Verification items for the finished model (mm, model axes). Face numbers are marked on the shaded views. A direction names the side the tool comes from. Give positions to 0.01 mm unless a question says otherwise; leave off trailing zeros. Write each loop counter-clockwise with the first axis right and the second up, starting at its lowest first coordinate (ties: lowest second). Pieces come first, ordered by that corner, then holes. Notation, with made-up numbers: M -8.75,-37.75 L 44.25,-37.75 A12 cw 44.25,-24.75 Z; hole C 6,-17.75 d11. An arc over 180 degrees is marked long. Answer as a JSON object with one key per item and string values.
```python
from build123d import *

# Parameters (mm, degrees)
SKETCH1_R                      = 6
BOSS_EXTRUDE1_DEPTH            = 2
SKETCH2_R                      = 3.95
BOSS_EXTRUDE2_DEPTH            = 7.9
CHAMFER1_SIZE                  = 0.4
CBORE_FOR_M3_SHCS1_D           = 3.2
CBORE_FOR_M3_SHCS1_CBORE_D     = 6
CBORE_FOR_M3_SHCS1_CBORE_DEPTH = 2.5


with BuildPart() as part:
    # Sketch1 → Boss-Extrude1 (new body)
    with BuildSketch(Plane(origin=(0, 0, 0), x_dir=(1, 0, 0), z_dir=(0, 1, 0))):
        Circle(SKETCH1_R)
    extrude(amount=BOSS_EXTRUDE1_DEPTH)

    # Sketch2 → Boss-Extrude2 (add)
    with BuildSketch(Plane(origin=(0, 2, 0), x_dir=(1, 0, 0), z_dir=(0, 1, 0))):
        Circle(SKETCH2_R)
    extrude(amount=BOSS_EXTRUDE2_DEPTH)

    # Chamfer1
    chamfer1_edges = [part.edges().sort_by_distance(p)[0] for p in [
        (-6, 0, 0),
        (-6, 2, 0),
        (-3.95, 9.9, 0),
    ]]
    chamfer(chamfer1_edges, length=CHAMFER1_SIZE)

    # CBORE for M3 SHCS1 (through all)
    with Locations(Plane(origin=(0, 0, 0), x_dir=(-1, 0, 0), z_dir=(0, -1, 0))):
        with Locations((0, 0)):
            CounterBoreHole(CBORE_FOR_M3_SHCS1_D / 2, CBORE_FOR_M3_SHCS1_CBORE_D / 2, CBORE_FOR_M3_SHCS1_CBORE_DEPTH)


solid = part.part
```
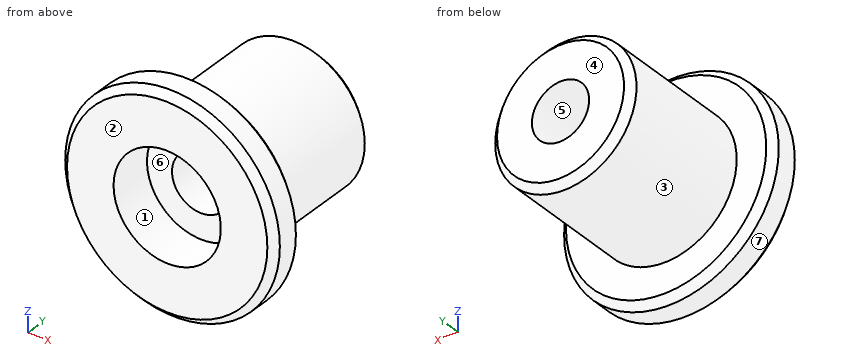
1) Access from +Z, -Z, +X, -X, +Y, -Y to the whole of each face (thin tool, end or side, straight path). Record for the marked faces 1, 2 and 3.
Completed:
{"face 1": "-Y", "face 2": "+Z, -Z, +X, -X, -Y", "face 3": "+Y"}
2) Section check D-D on y = 1.25. Record the boundary of the cut face in (x, z), and give its area (3 significant figures).
Completed:
{"outline": "C 0,0 d12; hole C 0,0 d6", "area": "84.8 mm2"}
3) Go/stop test with flat-tipped pins: pin 1 (2 mm diameter, centred on x = -4.5, y = 5.5, fed in from +Z); pin 2 (5 mm diameter, centred on y = 5.5, z = -1.5, fed in from +X); pin 3 (3 mm diameter, centred on x = -1, y = 6.5, fed in from -Z). Record where each tip stops, or that it passes through.
Completed:
{"pin 1": "stops at z = 1.83", "pin 2": "stops at x = 3.95", "pin 3": "stops at z = -3.95"}
4) Section check A-A on x = 0. Record the boundary of the cut face in (y, z).
Completed:
{"outline": "M 0,-5.6 L 0.4,-6 L 1.6,-6 L 2,-5.6 L 2,-3.95 L 9.5,-3.95 L 9.9,-3.55 L 9.9,-1.6 L 2.5,-1.6 L 2.5,-3 L 0,-3 Z; M 0,3 L 2.5,3 L 2.5,1.6 L 9.9,1.6 L 9.9,3.55 L 9.5,3.95 L 2,3.95 L 2,5.6 L 1.6,6 L 0.4,6 L 0,5.6 Z"}
5) Section check C-C on y = 5. Record the boundary of the cut face in (x, z).
Completed:
{"outline": "C 0,0 d7.9; hole C 0,0 d3.2"}
6) Section check B-B on z = 0. Record the boundary of the cut face in (x, y).
Completed:
{"outline": "M -6,0.4 L -5.6,0 L -3,0 L -3,2.5 L -1.6,2.5 L -1.6,9.9 L -3.55,9.9 L -3.95,9.5 L -3.95,2 L -5.6,2 L -6,1.6 Z; M 1.6,2.5 L 3,2.5 L 3,0 L 5.6,0 L 6,0.4 L 6,1.6 L 5.6,2 L 3.95,2 L 3.95,9.5 L 3.55,9.9 L 1.6,9.9 Z"}
7) Release check for a two-part mould opening along Z. For the marked faces 4, 5, 6 and 7 record: pulls with the +Z half, pulls with the -Z half, needs draft (parallel to the pull), parting line crosses it, or undercut.
Completed:
{"face 4": "needs draft", "face 5": "undercut", "face 6": "undercut", "face 7": "parting line crosses it"}
8) Thickness scan on L1, parallel to Z at x = 0, y = 0.75; L2, parallel to Y at x = -4, z = -2; L3, parallel to Z at x = -1.5, y = 1. Record the ranges inside material, lowest first.
Completed:
{"L1": "z = -6 to -3, 3 to 6", "L2": "y = 0 to 2", "L3": "z = -5.81 to -2.6, 2.6 to 5.81"}
